Geometry: see drawing. Coordinates: mm, zero at the bounding-box minimum. A direction names the side the tool comes from. Give positions to 0.01 mm unless a question says otherwise; leave off trailing zeros. Order: outer loops, then holes, each group sorted by start corner. A loop starts at its lowest first (then second) coordinate and runs counter-clockwise, first axis right, second up. Notation, with made-up numbers: (-34.75, -37) - (-27.75, -37) arc R16 cw to (-27.75, -19) - close; hole circle Ø9 at (41, 75.5). An arc over 180 degrees is marked (long way). Write item = value, one per line. Start each with the question number.
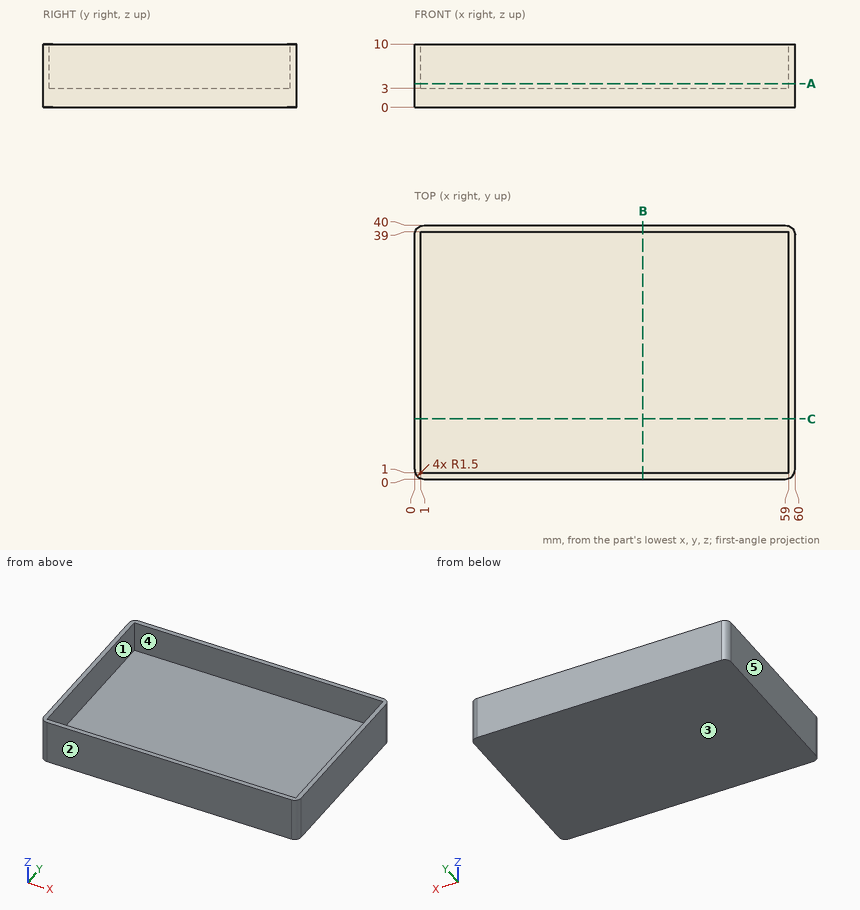
Q1. Material intervals for line 1 along X through (y, z) = (25.5, 8.25); line 2 along Y through (x, z) = (14, 6); line 3 along Z through (x, y) = (18.5, 20), sorted ascending. Write a range as from..to.
Q2. Section B-B, the plane x = 36. Return the cut outline in (y, z), then the cut area to 3 significant figures.
Q3. Set-up query: the marked faces 4 and 5. Return all of +Z, -Z, +X, -X, +Y, -Y with unobstructed straight access to the full face (end or side cutting, diameter ignored); none if empty.
Q4. Contact query for a flat-ended pin moving along its axis: pin 1 (8 mm diameter, centred on x = 26.5, y = 32.5, fed in from +Z). Output: stop coordinate, or through.
Q5. Pull-direction query (Y, two-part tool) for the marked faces 1, 2 and 3; classes: +Y half, -Y half, draft (parallel to the pull), parting line (faces both ways), or undercut.
Q6. Section A-A, the plane z = 3.75. Return the cut outline in (x, y), then the cut area to 3 significant figures.
Q7. Section C-C, the plane y = 9.5. Return the cut outline in (x, z), then the cut area to 3 significant figures.
The answers:
q1.line_1 = 0..1, 59..60
q1.line_2 = 0..1, 39..40
q1.line_3 = 0..3
q2.outline = (0, 0) - (40, 0) - (40, 10) - (39, 10) - (39, 3) - (1, 3) - (1, 10) - (0, 10) - close
q2.area = 134 mm²
q3.face_4 = +Z
q3.face_5 = +Z, -Z, -X, +Y, -Y
q4.pin_1 = 3
q5.face_1 = undercut
q5.face_2 = -Y half
q5.face_3 = draft
q6.outline = (0, 1.5) arc R1.5 ccw to (1.5, 0) - (58.5, 0) arc R1.5 ccw to (60, 1.5) - (60, 38.5) arc R1.5 ccw to (58.5, 40) - (1.5, 40) arc R1.5 ccw to (0, 38.5) - close; hole (1, 1) - (59, 1) - (59, 39) - (1, 39) - close
q6.area = 194 mm²
q7.outline = (0, 0) - (60, 0) - (60, 10) - (59, 10) - (59, 3) - (1, 3) - (1, 10) - (0, 10) - close
q7.area = 194 mm²
